Part model, mm, in its own coordinate system. Give positions to 0.01 mm unless a question says otherwise; leave off trailing zeros. Order: outer loops, then holes, each group sorted by start corner. A loop starts at its lowest first (then second) coordinate and runs counter-clockwise, first axis right, second up. Notation, with made-up numbers: M 44,12 L 71,12 A23 cw 71,48 Z; hole C 72.5,1 d11. An arc over 180 degrees is marked long. Answer as a JSON object with one key per item and string values.
Autodesk Inventor part; units mm, degrees
ref_plane "YZ Plane" through (0, 0, 0) normal (1, 0, 0) x (0, 1, 0)
ref_plane "XZ Plane" through (0, 0, 0) normal (0, 1, 0) x (-1, 0, 0)
ref_plane "XY Plane" through (0, 0, 0) normal (0, 0, 1) x (1, 0, 0)
sketch "Sketch1" plane through (0, 0, 0) normal (0, 0, 1) x (1, 0, 0)
  line L0 (0, 0) -> (0, 8.5)
  line L1 (0, 8.5) -> (3, 8.5)
  line L2 (3, 8.5) -> (3, 11.5)
  line L3 (3, 11.5) -> (0, 11.5)
  line L4 (0, 11.5) -> (0, 68.5)
  line L5 (0, 68.5) -> (3, 68.5)
  line L6 (3, 68.5) -> (3, 71.5)
  line L7 (3, 71.5) -> (0, 71.5)
  line L8 (0, 71.5) -> (0, 78)
  line L9 (-12, 0) -> (-12, -3)
  line L10 (-12, -3) -> (-9, -3)
  line L11 (-9, -3) -> (-9, 0)
  line L12 (-9, 0) -> (-3, 0)
  line L13 (-3, 0) -> (-3, -3)
  line L14 (-3, -3) -> (0, -3)
  line L15 (0, -3) -> (0, 0)
  line L16 (0, 78) -> (-5.5, 78)
  line L17 (-12, 0) -> (-12, 3)
  line L18 (-12, 3) -> (-5.5, 78)
  line L19 (-15, 0) -> (6, 0) construction
  line L20 (3, 10) -> (0, 10) construction
  line L21 (3, 70) -> (0, 70) construction
  line L22 (-4.3, 76.5) -> (-3, 76.5)
  line L23 (-3, 76.5) -> (-3, 73.5)
  line L24 (-3, 73.5) -> (-4.3, 73.5)
  line L25 (-4.3, 73.5) -> (-4.3, 76.5)
  line L26 (-4.3, 75) -> (-3, 75) construction
  line L27 (-7.5, 4.3) -> (-4.5, 4.3)
  line L28 (-4.5, 4.3) -> (-4.5, 3)
  line L29 (-4.5, 3) -> (-7.5, 3)
  line L30 (-7.5, 3) -> (-7.5, 4.3)
  line L31 (-6, 3) -> (-6, 0) construction
  line L32 (-4.3, 66.5) -> (-3, 66.5)
  line L33 (-3, 66.5) -> (-3, 63.5)
  line L34 (-3, 63.5) -> (-4.3, 63.5)
  line L35 (-4.3, 63.5) -> (-4.3, 66.5)
  line L36 (-4.3, 65) -> (-3, 65) construction
  line L37 (-4.3, 16.5) -> (-3, 16.5)
  line L38 (-3, 16.5) -> (-3, 13.5)
  line L39 (-3, 13.5) -> (-4.3, 13.5)
  line L40 (-4.3, 13.5) -> (-4.3, 16.5)
  line L41 (-4.3, 15) -> (-3, 15) construction
  line L42 (-3, 6.5) -> (-4.3, 6.5)
  line L43 (-4.3, 5) -> (-3, 5) construction
  line L44 (-3, 3.5) -> (-3, 6.5)
  line L45 (-4.3, 3.5) -> (-3, 3.5)
  line L46 (-4.3, 6.5) -> (-4.3, 3.5)
  line L47 (0, 50) -> (-3, 50) construction
  line L48 (-4.3, 53.5) -> (-3, 53.5)
  line L49 (-3, 53.5) -> (-3, 56.5)
  line L50 (-3, 56.5) -> (-4.3, 56.5)
  line L51 (-4.3, 56.5) -> (-4.3, 53.5)
  line L52 (-4.3, 55) -> (-3, 55) construction
  line L53 (-4.3, 46.5) -> (-3, 46.5)
  line L54 (-3, 46.5) -> (-3, 43.5)
  line L55 (-3, 43.5) -> (-4.3, 43.5)
  line L56 (-4.3, 43.5) -> (-4.3, 46.5)
  line L57 (-4.3, 45) -> (-3, 45) construction
  circle A0 centre (-5, 30) radius 1.85
  dimension "d0" = 3
  dimension "d1" = 12
  dimension "d2" = 3
  dimension "d3" = 10
  dimension "d4" = 60
  dimension "d5" = 5.5
  dimension "d6" = 3
  dimension "d7" = 1.3
  dimension "d8" = 3
  dimension "d9" = 5
  dimension "d10" = 3
  dimension "d11" = 1.3
  dimension "d12" = 3
  dimension "d13" = 3
  dimension "d14" = 3
  dimension "d15" = 1.3
  dimension "d16" = 5
  dimension "d17" = 3
  dimension "d18" = 1.3
  dimension "d19" = 5
  dimension "d29" = 5
  dimension "d30" = 50
  dimension "d31" = 3.7
  dimension "d32" = 5
  dimension "d33" = 30
extrude "Extrusion1" add sketch "Sketch1" along normal blind 3
fillet "Fillet1" radius 1 8 edges at (3, 11.5, 1.5) (3, 8.5, 1.5) (0, -3, 1.5) (-3, -3, 1.5) (-9, -3, 1.5) (-12, -3, 1.5) (3, 68.5, 1.5) (3, 71.5, 1.5)
fillet "Fillet2" radius 3 1 edges at (-5.5, 78, 1.5)
fillet "Fillet2" radius 20 1 edges at (-12, 3, 1.5)
chamfer "Chamfer1" distance 1 angle 45 14 edges at (-6, 3, 3) (-6, 3, 0) (-3, 15, 3) (-3, 15, 0) (-3, 65, 3) (-3, 65, 0) (-3, 75, 3) (-3, 75, 0) (-3, 5, 3) (-3, 5, 0) (-3, 45, 0) (-3, 45, 3) (-3, 55, 0) (-3, 55, 3)
properties part number "turtlebot_installation_fin_bottom"
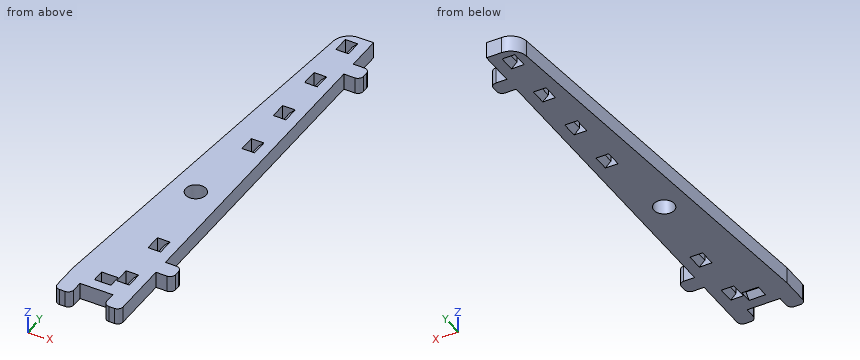
1. Cut at A-A on y = 30. Give the cut face in (x, z).
Worked answers:
{"outline": "M -9.66,0 L -6.85,0 L -6.85,3 L -9.66,3 Z; M -3.15,0 L 0,0 L 0,3 L -3.15,3 Z"}
2. Cut at B-B on y = 58. Give the cut face in (x, z).
Worked answers:
{"outline": "M -7.23,0 L 0,0 L 0,3 L -7.23,3 Z"}
3. Probe line 1 along Y through (x, z) = (2, 0.85); line 2 along Y through (x, z) = (-5, 0.95); line 3 along X through (y, z) = (29.5, 1.25). List the from-to ranges inside material, lowest first.
Worked answers:
{"line 1": "y = 8.5 to 11.5, 68.5 to 71.5", "line 2": "y = 0 to 2.95, 4.3 to 28.15, 31.85 to 76.98", "line 3": "x = -9.7 to -6.78, -3.22 to 0"}
4. Pin check, flat tips, straight feed: P1, Ø0.8, axis at y = 54.5, z = 1.5, coming from the -X side; P2, Ø0.7, axis at x = -3, z = 1.5, coming from the -Y side; P3, Ø0.8, axis at y = 4.5, z = 1.5, coming from the -X side. Stop position of each tip, or through.
Worked answers:
{"P1": "stops at x = -7.57", "P2": "stops at y = -2.76", "P3": "stops at x = -11.9"}
